Verification items for the finished model (mm, model axes). A direction names the side the tool comes from. Round coordinates to 2 decimals unless told otherwise and drop trailing zeros. Loops run counter-clockwise (first coordinate to the right, second up) from the corner with the lowest first, then second, coordinate; pieces in that order, holes last. Notation, with made-up numbers: (84, 58.25) -> (119, 58.25) arc R11 ccw to (119, 72.25) -> close; hole circle Ø5 at (-23, 82). An arc over 180 degrees is marked (long way). Write item = value, one per line.
```python
from build123d import *

# Parameters (mm, degrees)
SKETCH_1_W          = 40
SKETCH_1_H          = 25
EXTRUDE_1_DEPTH     = 99
SKETCH_2_R          = 14
CUT_EXTRUDE_1_DEPTH = 110.66312051
SKETCH_3_W          = 46
SKETCH_3_H          = 46
EXTRUDE_2_DEPTH     = 10
SKETCH_4_R          = 1.6
CUT_EXTRUDE_2_DEPTH = 10
SKETCH_5_R          = 3
CUT_EXTRUDE_3_DEPTH = 4
FILLET_1_R          = 3
SKETCH_6_R          = 1.5
CUT_EXTRUDE_4_DEPTH = 10


with BuildPart() as part:
    # 草图1 → 凸台-拉伸1 (new body)
    with BuildSketch(Plane(origin=(0, 0, 0), x_dir=(0, 0, -1), z_dir=(1, 0, 0))):
        with Locations((20, -12.5)):
            Rectangle(SKETCH_1_W, SKETCH_1_H)
    extrude(amount=EXTRUDE_1_DEPTH)

    # 草图2 → 切除-拉伸1 (cut, through all)
    with BuildSketch(Plane.ZY):
        with Locations((-20, 3.5)):
            Circle(SKETCH_2_R)
    extrude(amount=-CUT_EXTRUDE_1_DEPTH, mode=Mode.SUBTRACT)

    # 草图3 → 凸台-拉伸2 (add)
    with BuildSketch(Plane(origin=(0, -25, 0), x_dir=(-1, 0, 0), z_dir=(0, -1, 0))):
        with Locations((-122, 20)):
            Rectangle(SKETCH_3_W, SKETCH_3_H)
    extrude(amount=-EXTRUDE_2_DEPTH)

    # 草图4 → 切除-拉伸2 (cut)
    with BuildSketch(Plane(origin=(0, -25, 0), x_dir=(-1, 0, 0), z_dir=(0, -1, 0))):
        with Locations(Location((-103.5, 1.5, 0), (0, 0, 90))):
            Circle(SKETCH_4_R)
        with Locations(Location((-140.5, 1.5, 0), (0, 0, 90))):
            Circle(SKETCH_4_R)
        with Locations(Location((-103.5, 38.5, 0), (0, 0, 90))):
            Circle(SKETCH_4_R)
        with Locations(Location((-140.5, 38.5, 0), (0, 0, 90))):
            Circle(SKETCH_4_R)
    extrude(amount=-CUT_EXTRUDE_2_DEPTH, mode=Mode.SUBTRACT)

    # 草图5 → 切除-拉伸3 (cut)
    with BuildSketch(Plane(origin=(0, -25, 0), x_dir=(-1, 0, 0), z_dir=(0, -1, 0))):
        with Locations(Location((-103.5, 1.5, 0), (0, 0, 90))):
            Circle(SKETCH_5_R)
        with Locations(Location((-103.5, 38.5, 0), (0, 0, 90))):
            Circle(SKETCH_5_R)
        with Locations(Location((-140.5, 38.5, 0), (0, 0, 90))):
            Circle(SKETCH_5_R)
        with Locations(Location((-140.5, 1.5, 0), (0, 0, 90))):
            Circle(SKETCH_5_R)
    extrude(amount=-CUT_EXTRUDE_3_DEPTH, mode=Mode.SUBTRACT)

    # 圆角1
    fillet_1_edges = [part.edges().sort_by_distance(p)[0] for p in [
        (99, -20, -40),
        (99, -20, 0),
    ]]
    fillet(fillet_1_edges, radius=FILLET_1_R - 0.0001)  # a hair under: the kernel refuses the full size

    # 草图6 → 切除-拉伸4 (cut)
    with BuildSketch(Plane(origin=(0, 0, 0), x_dir=(1, 0, 0), z_dir=(0, 1, 0))):
        with Locations(Location((49.5, 36.777720856, 0), (0, 0, 270))):
            Circle(SKETCH_6_R)
        with Locations(Location((49.5, 3.222279144, 0), (0, 0, 270))):
            Circle(SKETCH_6_R)
        with Locations(Location((19.5, 36.777720856, 0), (0, 0, 270))):
            Circle(SKETCH_6_R)
        with Locations(Location((19.5, 3.222279144, 0), (0, 0, 270))):
            Circle(SKETCH_6_R)
        with Locations(Location((79.5, 36.777720856, 0), (0, 0, 270))):
            Circle(SKETCH_6_R)
        with Locations(Location((79.5, 3.222279144, 0), (0, 0, 270))):
            Circle(SKETCH_6_R)
    extrude(amount=-CUT_EXTRUDE_4_DEPTH, mode=Mode.SUBTRACT)


solid = part.part
```
(1) Sectioned sample at A-A, the plane x = 140.5. Record the cut outline in (y, z), and give its area (3 significant figures).
Filled sheet:
outline = (-25, -43) -> (-15, -43) -> (-15, -40.1) -> (-21, -40.1) -> (-21, -41.5) -> (-25, -41.5) -> close; (-25, -35.5) -> (-21, -35.5) -> (-21, -36.9) -> (-15, -36.9) -> (-15, -3.1) -> (-21, -3.1) -> (-21, -4.5) -> (-25, -4.5) -> close; (-25, 1.5) -> (-21, 1.5) -> (-21, 0.1) -> (-15, 0.1) -> (-15, 3) -> (-25, 3) -> close
area = 374 mm2
(2) Draft check along X on faces 1 (the face through (98.14, -19.93, -40.9)), 2 (the face through (143.03, -23.03, -3.11)), 3 (the face through (74, -25, -20)). Enter one of: released by +X, released by -X, zero draft, split by the parting line, or undercut.
Filled sheet:
face_1 = released by -X
face_2 = undercut
face_3 = zero draft
(3) Go/stop test with flat-tipped pins: pin 1 Ø8 at (x, y) = (67, -15.5) entering from -Z; pin 2 Ø3 at (y, z) = (-8.5, -10.5) entering from +X; pin 3 Ø1 at (x, z) = (97, -27.5) entering from +Y. Record where each tip stops, or that it passes through.
Filled sheet:
pin_1 = -40
pin_2 = 99
pin_3 = -7.99
(4) Set-up check for faces 4 (the face through (20, -10, -37)), 5 (the face through (99, -11, -20)), 6 (the face through (138.94, -18.04, -1.15)), 7 (the face through (145, -20, -20)), 8 (the face through (102, -21, -40)): record each of +Z, -Z, +X, -X, +Y, -Y from which the full face is reachable in a straight line by a thin tool's end or side.
Filled sheet:
face_4 = +Y
face_5 = +Z, -Z, +X, +Y
face_6 = +Y, -Y
face_7 = +Z, -Z, +X, +Y, -Y
face_8 = -Y
(5) Sectioned sample at B-B, the plane y = -8. Record the cut outline in (x, z).
Filled sheet:
outline = (0, -40) -> (99, -40) -> (99, -27.98) -> (0, -27.98) -> close; (0, -12.02) -> (99, -12.02) -> (99, 0) -> (0, 0) -> close; hole circle Ø3 at (19.5, -36.78); hole circle Ø3 at (19.5, -3.22); hole circle Ø3 at (49.5, -36.78); hole circle Ø3 at (49.5, -3.22); hole circle Ø3 at (79.5, -36.78); hole circle Ø3 at (79.5, -3.22)
(6) Sectioned sample at C-C, the plane y = -19. Count the separate pieces of the cut face and the enclosed holes in it, and give its area (3 significant figures).
Filled sheet:
separate_pieces = 1
enclosed_holes = 4
area = 6,050 mm2
(7) Sectioned sample at D-D, the plane x = 19.5. Record the cut outline in (y, z).
Filled sheet:
outline = (-25, -40) -> (0, -40) -> (0, -38.28) -> (-10, -38.28) -> (-10, -35.28) -> (0, -35.28) -> (0, -33.56) arc R14 cw to (0, -6.44) -> (0, -4.72) -> (-10, -4.72) -> (-10, -1.72) -> (0, -1.72) -> (0, 0) -> (-25, 0) -> close
(8) Material ranges on probe 1 along X at (y, z) = (-16.65, -1.5); probe 2 along Z at (x, y) = (79.5, -4.75); probe 3 along X at (y, z) = (-21.5, -4), recorded low to high. Write a range as from..to.
Filled sheet:
probe_1 = 0..101.9, 105.1..138.9, 142.1..145
probe_2 = -40..-38.28, -35.28..-31.31, -8.69..-4.72, -1.72..0
probe_3 = 0..101.84, 105.16..138.84, 142.16..145
